```python
from build123d import *

# Parameters (mm, degrees)
F0_W     = 101.186872
F0_H     = 81.592738
F1_DEPTH = 25.4
F2_SIZE  = 5.08
F3_SIZE  = 5.08
F4_R     = 7.62


with BuildPart() as f1:
    # F0 (on Top) → F1 (new body)
    with BuildSketch(Plane.XY):
        Rectangle(F0_W, F0_H)
    extrude(amount=F1_DEPTH)

    # F2
    f2_edges = [f1.edges().sort_by_distance(p)[0] for p in [
        (0, -40.796369, 0),
        (-50.593436, 0, 0),
        (0, 40.796369, 0),
        (50.593436, 0, 0),
    ]]
    chamfer(f2_edges, length=F2_SIZE)

    # F3
    f3_edges = [f1.edges().sort_by_distance(p)[0] for p in [
        (0, -40.796369, 25.4),
        (50.593436, 0, 25.4),
        (0, 40.796369, 25.4),
        (-50.593436, 0, 25.4),
    ]]
    chamfer(f3_edges, length=F3_SIZE)

    # F4
    f4_edges = [f1.edges().sort_by_distance(p)[0] for p in [
        (-50.593436, -40.796369, 12.7),
        (-50.593436, 40.796369, 12.7),
        (50.593436, 40.796369, 12.7),
        (50.593436, -40.796369, 12.7),
    ]]
    fillet(f4_edges, radius=F4_R)


solid = f1.part
```
Model file for the job. Use its own axes, mm. Coordinates: 2 decimals unless noted, no trailing zeros. Order: outer loops, then holes, each group sorted by start corner. A loop starts at its lowest first (then second) coordinate and runs counter-clockwise, first axis right, second up. Notation, with made-up numbers: (-35.5, 87) - (14.5, 87) arc R10 cw to (14.5, 93) - close; hole circle Ø8 at (53.25, 44). An arc over 180 degrees is marked (long way). Return JSON: item names as keys, results as strings. Group by question number.
1) Flat gauge pin, fed straight in: P1, Ø2, axis at y = -23.5, z = 22, coming from the +X side. Where does the tip first touch, or does it go through?
2) Saw through at B-B, the plane y = 4. Write the cut outline in (x, z).
3) Probe line 1 (X direction, y = -35, z = 21.25); line 2 (Y direction, x = 26.5, z = 22.5); line 3 (X direction, y = 36, z = 24.5). List the from-to ranges inside material, lowest first. Write a range as from..to.
4) Saw through at A-A, the plane x = -28.5. Write the cut outline in (y, z), plus the area to 3 significant figures.
Values found:
{
 "1": {"P1": "stops at x = 49.91"},
 "2": {"outline": "(-50.59, 5.08) - (-45.51, 0) - (45.51, 0) - (50.59, 5.08) - (50.59, 20.32) - (45.51, 25.4) - (-45.51, 25.4) - (-50.59, 20.32) - close"},
 "3": {"line 1": "x = -49.66..49.66", "line 2": "y = -38.62..38.62", "line 3": "x = -46.41..46.41"},
 "4": {"outline": "(-40.8, 5.08) - (-35.72, 0) - (35.72, 0) - (40.8, 5.08) - (40.8, 20.32) - (35.72, 25.4) - (-35.72, 25.4) - (-40.8, 20.32) - close", "area": "2,020 mm²"}
}
